```python
from build123d import *

# Parameters (mm, degrees)
BOSS_EXTRUDE1_DEPTH = 8


with BuildPart() as part:
    # Sketch1 → Boss-Extrude1 (new body)
    with BuildSketch(Plane.XY):
        with BuildLine():
            Line((12, 14), (18, 14))
            ThreePointArc((18, 14), (19.414213562, 14.585786438), (20, 16))
            Line((20, 16), (20, 22))
            ThreePointArc((20, 22), (19.414213562, 23.414213562), (18, 24))
            Line((18, 24), (-18, 24))
            ThreePointArc((-18, 24), (-19.414213562, 23.414213562), (-20, 22))
            Line((-20, 22), (-20, 16))
            ThreePointArc((-20, 16), (-19.414213562, 14.585786438), (-18, 14))
            Line((-18, 14), (-12, 14))
            ThreePointArc((-12, 14), (-10.585786438, 13.414213562), (-10, 12))
            Line((-10, 12), (-10, -6))
            ThreePointArc((-10, -6), (-9.414213562, -7.414213562), (-8, -8))
            Line((-8, -8), (10, -8))
            Line((10, -8), (10, -1))
            Line((10, -1), (5.408326913, -1))
            ThreePointArc((5.408326913, -1), (-5.5, 0), (5.408326913, 1))
            Line((5.408326913, 1), (10, 1))
            Line((10, 1), (10, 12))
            ThreePointArc((10, 12), (10.585786438, 13.414213562), (12, 14))
        make_face()
    extrude(amount=BOSS_EXTRUDE1_DEPTH)


solid = part.part
```
Read the model definition and answer for the solid it produces. Units are mm, in the model's axes. A direction names the side the tool comes from. Round coordinates to 2 decimals unless told otherwise and drop trailing zeros. Write each loop counter-clockwise with the first axis right and the second up, starting at its lowest first coordinate (ties: lowest second). Pieces come first, ordered by that corner, then holes. Notation, with made-up numbers: M 39.25,29 L 66.25,29 A27 cw 66.25,64 Z; hole C -8,7 d9. An arc over 180 degrees is marked long. One line per item, written item: value.
Q1. Find section A-A on x = -1. Write down the section's boundary in (y, z), plus the area to 3 significant figures.
Data:
outline: M -8,0 L -5.41,0 L -5.41,8 L -8,8 Z; M 5.41,0 L 24,0 L 24,8 L 5.41,8 Z
area: 169 mm2
Q2. For a pull along Y with two mould halves and no side action, classify faces 6 (the cylindrical face through (-19.43, 14.6, 3.94)), 7 (the flat face through (-20, 19, 4)), 8 (the cylindrical face through (-5.495, -0.228, 3.944)) as +Y half, -Y half, draft (parallel to the pull), parting line (faces both ways), or undercut.
Data:
face 6: -Y half
face 7: draft
face 8: undercut
Q3. Flat-ended cylindrical pins translate along their axes: pin 1 Ø3.5 at (y, z) = (-6, 4) entering from +X; pin 2 Ø1.8 at (x, z) = (16, 2) entering from -Y; pin 3 Ø4 at (y, z) = (4, 5) entering from -X. Find the tip coordinate at first contact, or state that the pin passes through.
Data:
pin 1: x = 10
pin 2: y = 14
pin 3: x = -10
Q4. Find section D-D on y = 7.5. Write down the section's boundary in (x, z).
Data:
outline: M -10,0 L 10,0 L 10,8 L -10,8 Z
Q5. Which of the six approach directions +Z, -Z, +X, -X, +Y, -Y give full straight-line access (tool end or side, diameter ignored) to faces 1 (the flat face through (8, 1, 4)), 2 (the flat face through (20, 19, 4)), 3 (the flat face through (0, 12, 0)), 4 (the flat face through (10, 6, 4)), 5 (the flat face through (-15, 14, 4))?
Data:
face 1: +Z, -Z, +X
face 2: +Z, -Z, +X, +Y, -Y
face 3: -Z, +X, -X, +Y, -Y
face 4: +Z, -Z, +X, -Y
face 5: +Z, -Z, -X, -Y
Q6. Find section B-B on y = 2.5. Write down the section's boundary in (x, z).
Data:
outline: M -10,0 L -4.9,0 L -4.9,8 L -10,8 Z; M 4.9,0 L 10,0 L 10,8 L 4.9,8 Z
Q7. Find section C-C on z = 2.75. Write down the section's boundary in (x, y).
Data:
outline: M -20,16 A2 ccw -18,14 L -12,14 A2 cw -10,12 L -10,-6 A2 ccw -8,-8 L 10,-8 L 10,-1 L 5.41,-1 A5.5 cw long 5.41,1 L 10,1 L 10,12 A2 cw 12,14 L 18,14 A2 ccw 20,16 L 20,22 A2 ccw 18,24 L -18,24 A2 ccw -20,22 Z
Q8. Straight lines are drawn through the part: line 1 (Y direction, x = 0, z = 5); line 2 (Y direction, x = 9.5, z = 1.75); line 3 (X direction, y = 11.5, z = 4.75). For each, find the intervals that lie inside material, in ascending order. Write a range as [from, to].
Data:
line 1: [-8, -5.5], [5.5, 24]
line 2: [-8, -1], [1, 24]
line 3: [-10, 10]
